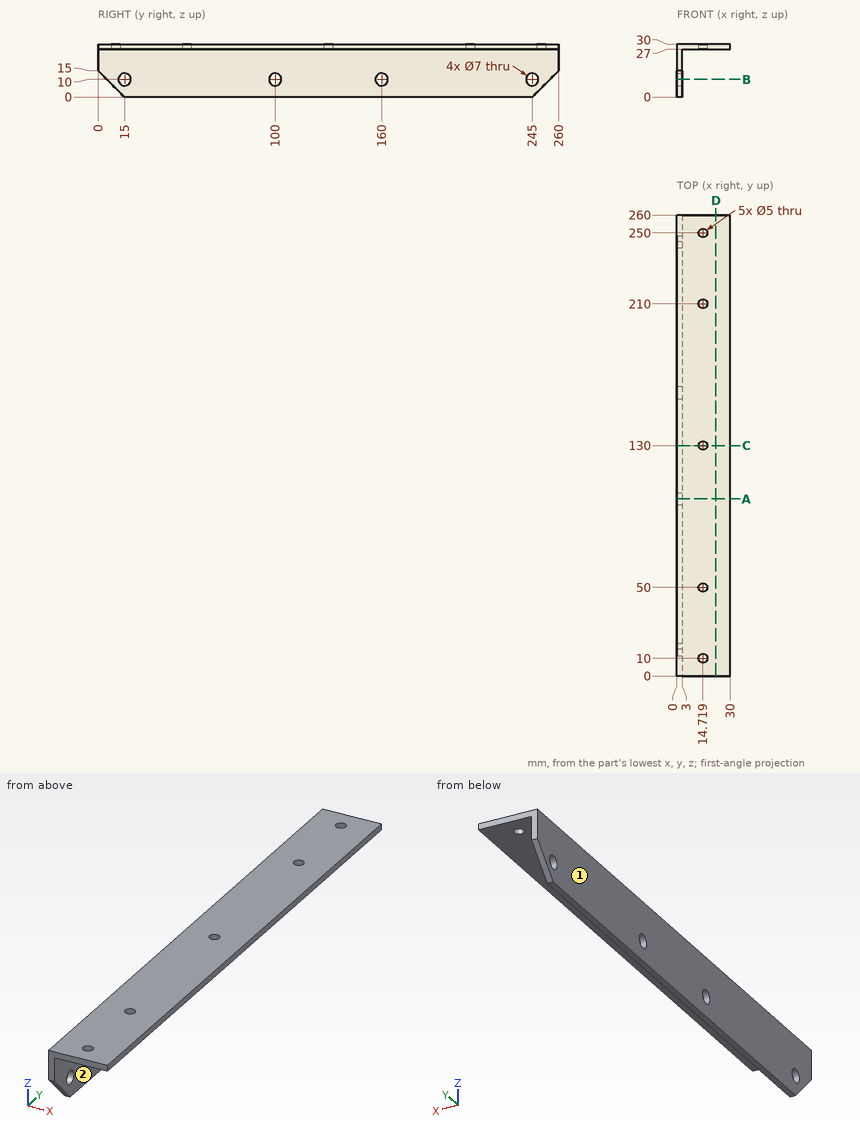
Geometry check sheet. Reference: drawing and pictorial views, mm from the part's lowest x, y, z. A direction names the side the tool comes from. Give positions to 0.01 mm unless a question says otherwise; leave off trailing zeros. Order: outer loops, then holes, each group sorted by start corner. A loop starts at its lowest first (then second) coordinate and runs counter-clockwise, first axis right, second up. Notation, with made-up numbers: M -1.5,22.25 L 26.5,22.25 A28 cw 26.5,57.25 Z; hole C 85.5,82 d7. An arc over 180 degrees is marked long. Return JSON: item names as keys, results as strings. Group by question number.
1) Section check C-C on y = 130. Record the cut outline in (x, z).
2) Section check B-B on z = 10. Record the cut outline in (x, y), and give its area (3 significant figures).
3) Scan lines: line 1 (Y direction, x = 2.5, z = 12.5); line 2 (Z direction, x = 1.2, y = 100); line 3 (X direction, y = 74.5, z = 24.5). Record each from-to range of solid material in increasing order.
4) Section check D-D on x = 22. Record the cut outline in (y, z).
5) Go/stop test with flat-tipped pins: pin 1 Ø8 at (x, y) = (14.72, 210) entering from -Z; pin 2 Ø8 at (y, z) = (55, 9.5) entering from +X. Record where each tip stops, or that it passes through.
6) Access from +Z, -Z, +X, -X, +Y, -Y to the whole of each face (thin tool, end or side, straight path). Record for the marked faces 1 and 2.
7) Section check A-A on y = 100. Record the cut outline in (x, z).
Answer block:
{
 "1": {"outline": "M 0,0 L 3,0 L 3,27 L 12.22,27 L 12.22,30 L 0,30 Z; M 17.22,27 L 30,27 L 30,30 L 17.22,30 Z"},
 "2": {"outline": "M 0,5 L 3,5 L 3,11.5 L 0,11.5 Z; M 0,18.5 L 3,18.5 L 3,96.5 L 0,96.5 Z; M 0,103.5 L 3,103.5 L 3,156.5 L 0,156.5 Z; M 0,163.5 L 3,163.5 L 3,241.5 L 0,241.5 Z; M 0,248.5 L 3,248.5 L 3,255 L 0,255 Z", "area": "666 mm^2"},
 "3": {"line 1": "y = 2.5 to 12.55, 17.45 to 97.55, 102.45 to 157.55, 162.45 to 242.55, 247.45 to 257.5", "line 2": "z = 0 to 6.5, 13.5 to 30", "line 3": "x = 0 to 3"},
 "4": {"outline": "M 0,27 L 260,27 L 260,30 L 0,30 Z"},
 "5": {"pin 1": "stops at z = 27", "pin 2": "stops at x = 3"},
 "6": {"face 1": "+Z, -Z, -X, +Y, -Y", "face 2": "-Z, +X, +Y, -Y"},
 "7": {"outline": "M 0,0 L 3,0 L 3,6.5 L 0,6.5 Z; M 0,13.5 L 3,13.5 L 3,27 L 30,27 L 30,30 L 0,30 Z"}
}
